Can you work these out from the model? Positions are in its coordinate system, mm. Face numbers are marked on the shaded views. Round coordinates to 2 decimals unless told otherwise and drop trailing zeros. Order: outer loops, then holes, each group sorted by start corner. A loop starts at its lowest first (then second) coordinate and runs counter-clockwise, first axis right, second up. Notation, with made-up numbers: (52.25, -18) -> (82.25, -18) arc R10 cw to (82.25, -13) -> close; hole circle Ø8 at (-34, -21). An arc over 180 degrees is marked (long way). One line per item, written item: value.
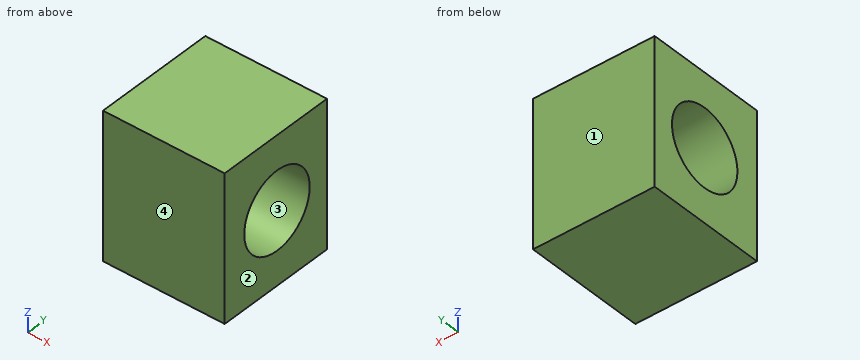
Autodesk Inventor part; units mm, degrees
ref_plane "YZ Plane" through (0, 0, 0) normal (1, 0, 0) x (0, 1, 0)
ref_plane "XZ Plane" through (0, 0, 0) normal (0, 1, 0) x (-1, 0, 0)
ref_plane "XY Plane" through (0, 0, 0) normal (0, 0, 1) x (1, 0, 0)
sketch "Sketch1" plane through (0, 0, 0) normal (1, 0, 0) x (0, 1, 0)
  line L0 (22.8278, 24.0961) -> (17.8278, 24.0961)
  line L1 (17.8278, 24.0961) -> (17.8278, 18.0961)
  line L2 (17.8278, 18.0961) -> (22.8278, 18.0961)
  line L3 (22.8278, 18.0961) -> (22.8278, 24.0961)
  point P0 (0, 0)
  dimension "d0" = 5
  dimension "d1" = 6
extrude "Extrusion1" add sketch "Sketch1" along normal blind 5
sketch "Sketch2" plane through (5, 0, 0) normal (1, 0, 0) x (0, 0, -1)
  point P0 (0, 0)
  point P1 (-21.0928, 20.384)
hole "Hole1" at (5, 20.384, 21.0928) direction (-1, 0, 0) diameter 3.2 end through all
properties part number "lcdholder"
Q1. I want a section at C-C on x = 2.55. List the corners of the cut face in (y, z) for me.
Answers below:
outline: (17.83, 18.1) -> (22.83, 18.1) -> (22.83, 24.1) -> (17.83, 24.1) -> close; hole circle Ø3.2 at (20.38, 21.09)
Q2. I want a section at B-B on y = 20.65. List the corners of the cut face in (x, z) for me, plus the area to 3 significant figures.
Answers below:
outline: (0, 18.1) -> (5, 18.1) -> (5, 19.52) -> (0, 19.52) -> close; (0, 22.67) -> (5, 22.67) -> (5, 24.1) -> (0, 24.1) -> close
area: 14.2 mm^2
Q3. Will this pin go through, and if not, where does the flat tip stop? pin 1 Ø1.5 at (y, z) = (20, 20) entering from -X.
Answers below:
pin 1: x = 0
Q4. I want a section at A-A on z = 21.1. List the corners of the cut face in (x, y) for me.
Answers below:
outline: (0, 17.83) -> (5, 17.83) -> (5, 18.78) -> (0, 18.78) -> close; (0, 21.98) -> (5, 21.98) -> (5, 22.83) -> (0, 22.83) -> close
Q5. Please list where these lines run through material, in increasing order: line 1 along Y through (x, z) = (2.05, 20.5); line 2 along Z through (x, y) = (1.4, 19.65); line 3 along Z through (x, y) = (2.6, 21.3).
Answers below:
line 1: 17.83 to 18.9, 21.87 to 22.83
line 2: 18.1 to 19.67, 22.51 to 24.1
line 3: 18.1 to 19.78, 22.4 to 24.1
Q6. We'd pull the mould along Y, two halves only. Please class the marked faces 1, 2, 3 and 4: released by +Y, released by -Y, zero draft, split by the parting line, or undercut.
Answers below:
face 1: released by +Y
face 2: zero draft
face 3: undercut
face 4: released by -Y
